```python
from build123d import *

# Parameters (mm, degrees)
PAD_DEPTH        = 8
SKETCH001_W      = 60
SKETCH001_H      = 5
PAD001_DEPTH     = 240
POCKET_DEPTH     = 5.001
POCKET001_DEPTH  = 5.001
PAD002_DEPTH     = 8
HOLE_D           = 4.4
HOLE_CSINK_D     = 8
HOLE_CSINK_ANGLE = 90


with BuildPart() as part:
    # Sketch → Pad (new body)
    with BuildSketch(Plane.XZ):
        with BuildLine():
            Line((-30, 0), (30, 0))
            Line((30, 0), (30, -23.38422))
            Line((30, -23.38422), (20.25, -23.38422))
            Line((20.25, -22.145781), (20.25, -23.38422))
            ThreePointArc((20.25, -22.145781), (14, -10.5), (7.75, -22.145781))
            Line((7.75, -22.145781), (7.75, -23.38422))
            Line((7.75, -23.38422), (-7.75, -23.38422))
            Line((-7.75, -22.145781), (-7.75, -23.38422))
            ThreePointArc((-7.75, -22.145781), (-14, -10.5), (-20.25, -22.145781))
            Line((-20.25, -22.145781), (-20.25, -23.38422))
            Line((-20.25, -23.38422), (-30, -23.38422))
            Line((-30, -23.38422), (-30, 0))
        make_face()
    extrude(amount=PAD_DEPTH)

    # Sketch001 (on Face14 of Pad) → Pad001 (join)
    with BuildSketch(Plane.XZ.offset(8)):
        with Locations((0, -2.5)):
            Rectangle(SKETCH001_W, SKETCH001_H)
    extrude(amount=PAD001_DEPTH)

    # Sketch002 (on Face15 of Pad001) → Pocket (cut, through all)
    with BuildSketch(Plane(origin=(0, 0, -5), x_dir=(1, 0, 0), z_dir=(0, 0, -1))):
        Polygon((-19.5, 251), (-33, 251), (-33, 0.857143), (-19.5, 33), align=None)
    extrude(amount=-POCKET_DEPTH, mode=Mode.SUBTRACT)

    # Sketch003 (on Face15 of Pocket) → Pocket001 (cut, through all)
    with BuildSketch(Plane(origin=(0, 0, -5), x_dir=(1, 0, 0), z_dir=(0, 0, -1))):
        Polygon((19.5, 251), (33, 251), (33, 0.857143), (19.5, 33), align=None)
    extrude(amount=-POCKET001_DEPTH, mode=Mode.SUBTRACT)

    # Sketch004 (on Face20 of Pocket001) → Pad002 (join)
    with BuildSketch(Plane.XZ.offset(248)):
        with BuildLine():
            Line((-19.5, 0), (19.5, 0))
            Line((19.5, 0), (19.5, -23.38422))
            Line((19.5, -23.38422), (18, -23.38422))
            Line((18, -20.38422), (18, -23.38422))
            ThreePointArc((18, -20.38422), (14, -13.822667), (10, -20.38422))
            Line((10, -20.38422), (10, -23.38422))
            Line((10, -23.38422), (-10, -23.38422))
            Line((-10, -20.38422), (-10, -23.38422))
            ThreePointArc((-10, -20.38422), (-14, -13.822667), (-18, -20.38422))
            Line((-18, -20.38422), (-18, -23.38422))
            Line((-18, -23.38422), (-19.5, -23.38422))
            Line((-19.5, -23.38422), (-19.5, 0))
        make_face()
    extrude(amount=-PAD002_DEPTH)

    # Hole (through all)
    with Locations(Plane(origin=(0, 0, -5), x_dir=(1, 0, 0), z_dir=(0, 0, -1))):
        with Locations((0, 30), (0, 130)):
            CounterSinkHole(HOLE_D / 2, HOLE_CSINK_D / 2, counter_sink_angle=HOLE_CSINK_ANGLE)


solid = part.part
```
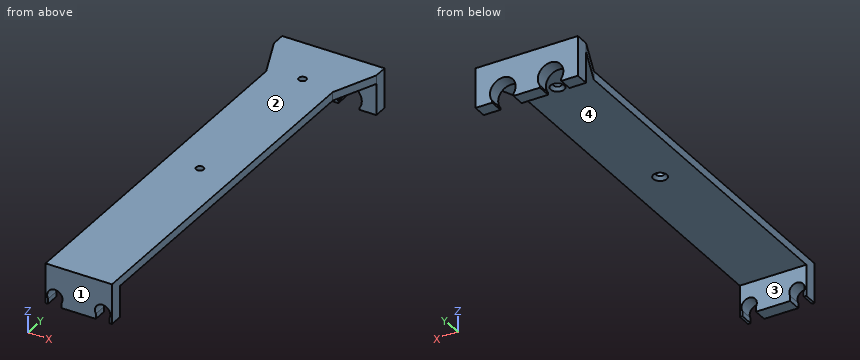
For this review, take the finished solid that the model builds, in its own axes (mm). Face numbers are marked on the shaded views. Round coordinates to 2 decimals unless told otherwise and drop trailing zeros. Write each loop counter-clockwise with the first axis right and the second up, starting at its lowest first coordinate (ties: lowest second). Pieces come first, ordered by that corner, then holes.
1) Take a section at B-B on y = -130. Give the boundary of the cut face in (x, z), then the cut area to 3 significant figures.
Answer below:
outline: (-19.5, -5) - (-4, -5) - (-2.2, -3.2) - (-2.2, 0) - (-19.5, 0) - close; (2.2, -3.2) - (4, -5) - (19.5, -5) - (19.5, 0) - (2.2, 0) - close
area: 170 mm2
2) Mouldability with a two-part tool opening along Y and no side actions: class the marked faces 1, 2, 3 and 4 as +Y half, -Y half, draft (parallel to the pull), parting line (faces both ways), or undercut.
Answer below:
face 1: -Y half
face 2: draft
face 3: undercut
face 4: undercut
3) Take a section at D-D on x = 14. Give the boundary of the cut face in (y, z), then the cut area to 3 significant figures.
Answer below:
outline: (-248, -13.82) - (-240, -13.82) - (-240, -5) - (-8, -5) - (-8, -10.5) - (0, -10.5) - (0, 0) - (-248, 0) - close
area: 1,350 mm2
4) Insertion check: pin 1 Ø7 at (y, z) = (-94, -7) entering from -X; pin 2 Ø7 at (x, y) = (0, -30) entering from -Z; pin 3 Ø2.5 at (y, z) = (-242.5, -22) entering from +X. Each pin has a flat end and moves straight along its axis. Give the tip position at first contact, or say it passes through.
Answer below:
pin 1: stops at x = -19.5
pin 2: stops at z = -4.5
pin 3: stops at x = 19.5
5) For line 1 along X through (y, z) = (-5.75, -18); line 2 along Y through (x, z) = (0, -1.65); line 3 along X through (y, z) = (-130, -1.95), list the stretches that pass through material, from the lowest coordinate up.
Answer below:
line 1: x = -30 to -21.5, -6.5 to 6.5, 21.5 to 30
line 2: y = -248 to -132.2, -127.8 to -32.2, -27.8 to 0
line 3: x = -19.5 to -2.2, 2.2 to 19.5
6) Take a section at A-A on x = 0. Give the boundary of the cut face in (y, z).
Answer below:
outline: (-248, -23.38) - (-240, -23.38) - (-240, -5) - (-134, -5) - (-132.2, -3.2) - (-132.2, 0) - (-248, 0) - close; (-127.8, -3.2) - (-126, -5) - (-34, -5) - (-32.2, -3.2) - (-32.2, 0) - (-127.8, 0) - close; (-27.8, -3.2) - (-26, -5) - (-8, -5) - (-8, -23.38) - (0, -23.38) - (0, 0) - (-27.8, 0) - close
7) Take a section at C-C on z = -18. Give the boundary of the cut face in (x, y), then the cut area to 3 significant figures.
Answer below:
outline: (-30, -8) - (-21.5, -8) - (-21.5, 0) - (-30, 0) - close; (-19.5, -248) - (-18.49, -248) - (-18.49, -240) - (-19.5, -240) - close; (-9.51, -248) - (9.51, -248) - (9.51, -240) - (-9.51, -240) - close; (-6.5, -8) - (6.5, -8) - (6.5, 0) - (-6.5, 0) - close; (18.49, -248) - (19.5, -248) - (19.5, -240) - (18.49, -240) - close; (21.5, -8) - (30, -8) - (30, 0) - (21.5, 0) - close
area: 408 mm2
